Study the drawing (mm; zero at the part's minimum x, y, z) and answer. A direction names the side the tool comes from. Give positions to 0.01 mm unless a question says otherwise; leave off trailing zeros. Order: outer loops, then holes, each group sorted by start corner. A loop starts at its lowest first (then second) coordinate and runs counter-clockwise, first axis right, second up.
Item 1: A cutting plane is placed at A-A (z = 97.5). Write down the section's boundary in (x, y).
Item 2: Which of the six approach directions +Z, -Z, +X, -X, +Y, -Y give full straight-line access (tool end or side, diameter ignored) to the marked faces 1, 2 and 3?
Item 3: A cutting plane is placed at D-D (y = 32). Write down the section's boundary in (x, z), plus the area to 3 significant figures.
Item 4: The mould has two halves that part along Z. Classify the marked faces 4, 5 and 6: +Z half, -Z half, draft (parallel to the pull), parting line (faces both ways), or undercut.
Item 5: Given pin 1 Ø2 at (x, y) = (143, 9) entering from -Z (3 decimals); pin 2 Ø5 at (y, z) = (48.5, 40) entering from +X; pin 3 Ø10 at (y, z) = (23, 43) entering from -X; pin 4 Ø2 at (x, y) = (23.5, 68.5) entering from +Z, each flat-ended and moving along its own axis, determine where each tip first touches the part or whether it passes through.
Item 6: A cutting plane is placed at B-B (y = 15). Write down the section's boundary in (x, z).
Item 7: Find the intervals of material crossed by line 1 along X through (y, z) = (69, 60.5); line 2 along Z through (x, y) = (21, 22); line 3 along Y through (x, z) = (24.5, 96.5), in increasing order.
Item 8: A cutting plane is placed at C-C (x = 152.5). Write down the section's boundary in (y, z).
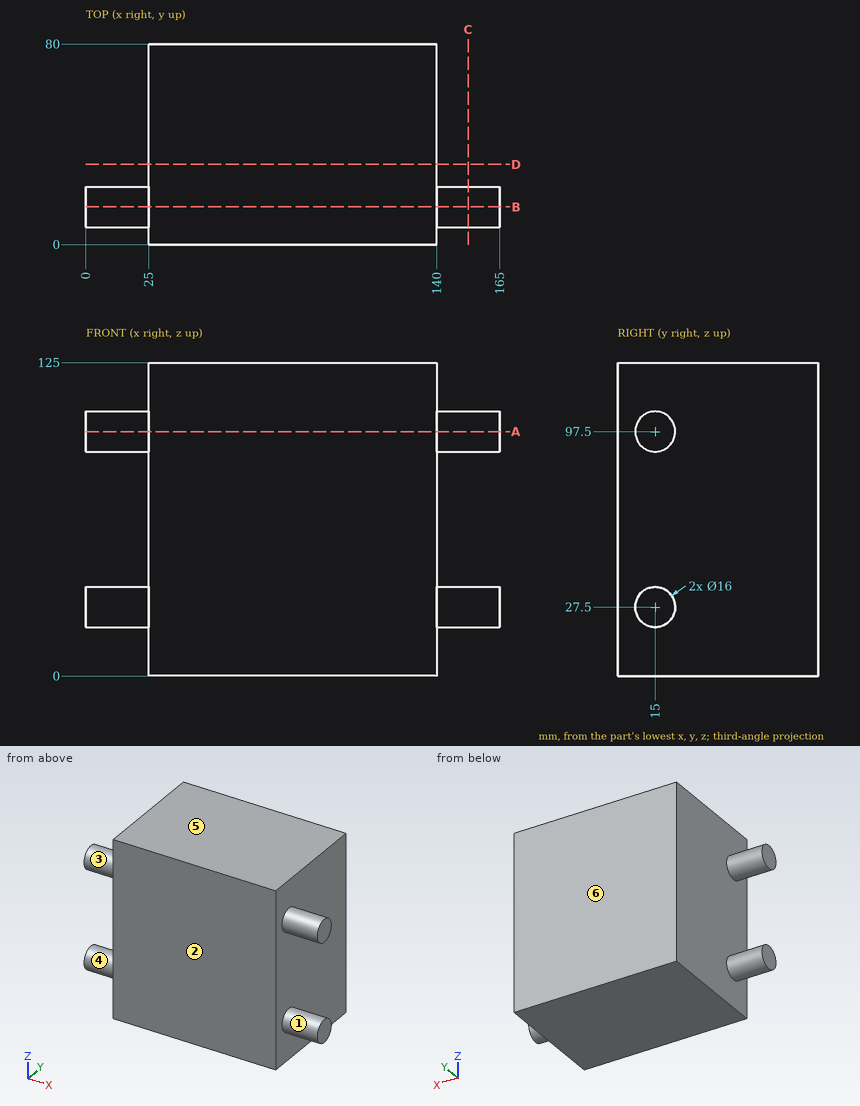
Response values:
1. outline: (0, 7) - (25, 7) - (25, 0) - (140, 0) - (140, 7) - (165, 7) - (165, 23) - (140, 23) - (140, 80) - (25, 80) - (25, 23) - (0, 23) - close
2. face 1: +X
2. face 2: +Z, -Z, +X, -X, -Y
2. face 3: -X
3. outline: (25, 0) - (140, 0) - (140, 125) - (25, 125) - close
3. area: 14,400 mm2
4. face 4: undercut
4. face 5: +Z half
4. face 6: draft
5. pin 1: stops at z = 21.255
5. pin 2: stops at x = 140
5. pin 3: stops at x = 25
5. pin 4: passes through
6. outline: (0, 19.5) - (25, 19.5) - (25, 0) - (140, 0) - (140, 19.5) - (165, 19.5) - (165, 35.5) - (140, 35.5) - (140, 89.5) - (165, 89.5) - (165, 105.5) - (140, 105.5) - (140, 125) - (25, 125) - (25, 105.5) - (0, 105.5) - (0, 89.5) - (25, 89.5) - (25, 35.5) - (0, 35.5) - close
7. line 1: x = 25 to 140
7. line 2: z = 23.63 to 31.37, 93.63 to 101.37
7. line 3: y = 7.06 to 22.94
8. outline: circle Ø16 at (15, 27.5); circle Ø16 at (15, 97.5)
